from build123d import *

# Parameters (mm, degrees)
F1_DEPTH  = 12.7
F6_DEPTH  = 12.7
F7_R      = 2.54
F8_DEPTH  = 12.7
F9_W      = 5.08
F9_H      = 2.54
F10_DEPTH = 6.35
F11_R     = 1.905
F12_DEPTH = 2.54
F14_DEPTH = 2.54


with BuildPart() as f1:
    # F0 (on Front) → F1 (new body)
    with BuildSketch(Plane.XZ):
        with BuildLine():
            ThreePointArc((-36.6009683429, 0), (-36.9808067883, 3.2622689922), (-38.1, 6.35))
            ThreePointArc((-38.1, 6.35), (-64.9990316571, 0), (-38.1, -6.35))
            ThreePointArc((-38.1, -6.35), (-36.9808067883, -3.2622689922), (-36.6009683429, 0))
        make_face()
    extrude(amount=F1_DEPTH)

    # F4 (on offset) → F5 (revolve, cut)
    with BuildSketch(Plane.XZ.offset(15.24)):
        with BuildLine():
            ThreePointArc((-63.5, 0), (-50.8, -12.7), (-38.1, 0))
            Line((-38.1, 0), (-63.5, 0))
        make_face()
    revolve(axis=Axis((-49.9650985003, -15.24, 0), (1, 0, 0)), mode=Mode.SUBTRACT)

    # F0 (on Front) → F6 (join)
    with BuildSketch(Plane.XZ):
        with BuildLine():
            Line((38.1, -6.35), (38.1, 6.35))
            Line((38.1, 6.35), (-38.1, 6.35))
            ThreePointArc((-38.1, 6.35), (-36.9808067883, 3.2622689922), (-36.6009683429, 0))
            ThreePointArc((-36.6009683429, 0), (-36.9808067883, -3.2622689922), (-38.1, -6.35))
            Line((-38.1, -6.35), (38.1, -6.35))
        make_face()
    extrude(amount=F6_DEPTH)

    # F7 (on face) → F8 (cut)
    with BuildSketch(Plane.XY.offset(6.35)):
        with Locations((31.75, -6.35)):
            Circle(F7_R)
    extrude(amount=-F8_DEPTH, mode=Mode.SUBTRACT)

    # F9 (on face) → F10 (join)
    with BuildSketch(Plane.XZ):
        with Locations((-52.2990316571, 0)):
            Rectangle(F9_W, F9_H)
    extrude(amount=-F10_DEPTH)

    # F11 (on face) → F12 (cut)
    with BuildSketch(Plane(origin=(0, 0, -1.27), x_dir=(1, 0, 0), z_dir=(0, 0, -1))):
        with Locations((-52.2990316571, -3.175)):
            Circle(F11_R)
    extrude(amount=-F12_DEPTH, mode=Mode.SUBTRACT)

    # F13 (on face) → F14 (join)
    with BuildSketch(Plane.XZ):
        Polygon((-36.6009683429, 0), (-36.6009683429, -6.35), (-34.0609683429, -6.35), (-34.0609683429, 6.35), (-36.6009683429, 6.35), align=None)
    extrude(amount=-F14_DEPTH)


solid = f1.part
Check sheet for the modelled part. Datum: model origin and axes. Units: mm. A direction names the side the tool comes from. Round coordinates to 2 decimals unless told otherwise and drop trailing zeros. Write each loop counter-clockwise with the first axis right and the second up, starting at its lowest first coordinate (ties: lowest second). Pieces come first, ordered by that corner, then holes. Notation, with made-up numbers: (41.5, 0) - (61.5, 0) arc R16 ccw to (61.5, 9) - close; hole circle Ø7 at (61.5, 79). An arc over 180 degrees is marked (long way). Return JSON: item names as keys, results as strings.
Q1. Cross-section at D-D (z = -11). Record the boundary of the cut face in (x, y), then the cut area to 3 significant figures.
Returned:
{"outline": "(-59.78, -12.7) - (-56.62, -12.7) arc R6.35 cw to (-44.98, -12.7) - (-41.82, -12.7) - (-41.82, 0) - (-59.78, 0) - close", "area": "196 mm²"}
Q2. Cross-section at C-C (z = 3.75). Record the boundary of the cut face in (x, y).
Returned:
{"outline": "(-64.49, -12.7) - (-62.66, -12.7) arc R12.13 cw to (-38.94, -12.7) - (38.1, -12.7) - (38.1, 0) - (-34.06, 0) - (-34.06, 2.54) - (-36.6, 2.54) - (-36.6, 0) - (-64.49, 0) - close; hole circle Ø5.08 at (31.75, -6.35)"}
Q3. Draft check along Y on faces 5 (the flat face through (-36.601, 1, 0)), 6 (the cylindrical face through (-50.482, 2.603, -0.018)), 7 (the cylindrical face through (31.2, -8.83, 0.09)), 8 (the flat face through (2, 0, 0)). Enter one of: released by +Y, released by -Y, zero draft, split by the parting line, or undercut.
Returned:
{"face 5": "zero draft", "face 6": "undercut", "face 7": "undercut", "face 8": "released by +Y"}
Q4. Depth check by flat-ended pin: P1, Ø8, axis at x = 2.5, y = 3, coming from the -Z side; P2, Ø6, axis at x = 13.5, y = -5, coming from the -Z side; P3, Ø3, axis at y = 3, z = 0.5, coming from the +X side. Enter the tip coordinate at first touch or a pass-through.
Returned:
{"P1": "stops at z = -6.35", "P2": "stops at z = -6.35", "P3": "stops at x = -34.06"}
Q5. Cross-section at B-B (y = -6.35). Record the boundary of the cut face in (x, z), then the cut area to 3 significant figures.
Returned:
{"outline": "(-38.1, -6.35) - (29.21, -6.35) - (29.21, 6.35) - (-38.1, 6.35) arc R14.2 ccw (long way) to start; (34.29, -6.35) - (38.1, -6.35) - (38.1, 6.35) - (34.29, 6.35) - close; hole circle Ø18.14 at (-50.8, 0)", "area": "1,270 mm²"}
Q6. Access from +Z, -Z, +X, -X, +Y, -Y to the whole of each face (thin tool, end or side, straight path). Record for faces 1 (the flat face through (-52, 1, -1.27)), 2 (the flat face through (-1, -7, -6.35)), 3 (the flat face through (1, -7, 6.35)), 4 (the flat face through (-52, 1, 1.27)).
Returned:
{"face 1": "-Z, -X, +Y", "face 2": "-Z, +X, +Y, -Y", "face 3": "+Z, +X, +Y, -Y", "face 4": "+Z, -X, +Y"}
Q7. Scan lines: L1, parallel to Y at x = 31.75, z = 1.5; L2, parallel to X at y = -6.25, z = 4.75; L3, parallel to X at y = -4.5, z = -1.5. Record each from-to range of solid material in increasing order. Write a range as from..to.
Returned:
{"L1": "y = -12.7..-8.89, -3.81..0", "L2": "x = -64.18..-58.41, -43.19..29.21, 34.29..38.1", "L3": "x = -64.92..-57.41, -44.19..30.01, 33.49..38.1"}
Q8. Cross-section at A-A (x = 31.75). Record the boundary of the cut face in (y, z), then the cut area to 3 significant figures.
Returned:
{"outline": "(-12.7, -6.35) - (-8.89, -6.35) - (-8.89, 6.35) - (-12.7, 6.35) - close; (-3.81, -6.35) - (0, -6.35) - (0, 6.35) - (-3.81, 6.35) - close", "area": "96.8 mm²"}
